from build123d import *

# Parameters (mm, degrees)
EXTRUDE_1_DEPTH             = 112
CUT_EXTRUDE_2_DEPTH         = 122.893396048
HOLE_WIZARD_M61_D           = 6.6
HOLE_WIZARD_M61_DEPTH       = 20
HOLE_WIZARD_M61_CBORE_D     = 11
HOLE_WIZARD_M61_CBORE_DEPTH = 12.4
HOLE_WIZARD_M61_TIP         = 1.982840043


with BuildPart() as part:
    # Эскиз1 → Бобышка-Вытянуть1 (new, symmetric)
    with BuildSketch(Plane.XY):
        Polygon((22.5, 0), (-22.5, 0), (-22.5, 10.4), (-7.5, 10.4), (-7.5, 17), (7.5, 17), (7.5, 10.4), (22.5, 10.4), align=None)
    extrude(amount=EXTRUDE_1_DEPTH, both=True)

    # Эскиз5 → Вырез-Вытянуть2 (cut, through all)
    with BuildSketch(Plane(origin=(22.5, 0, 0), x_dir=(0, 0, -1), z_dir=(1, 0, 0))):
        Polygon((-112, 0), (-48.555136271, 17), (-112, 17), align=None)
    extrude(amount=-CUT_EXTRUDE_2_DEPTH, mode=Mode.SUBTRACT)

    # Цековка для винта с внутренним шестигранником M61
    with Locations(Plane(origin=(0, 17, 0), x_dir=(1, 0, 0), z_dir=(0, 1, 0))):
        with Locations((0, -210), (0, 70), (0, -70)):
            CounterBoreHole(HOLE_WIZARD_M61_D / 2, HOLE_WIZARD_M61_CBORE_D / 2, HOLE_WIZARD_M61_CBORE_DEPTH, depth=HOLE_WIZARD_M61_DEPTH)
            with Locations((0, 0, -(HOLE_WIZARD_M61_DEPTH + HOLE_WIZARD_M61_TIP / 2))):  # 118° drill point
                Cone(0, HOLE_WIZARD_M61_D / 2, HOLE_WIZARD_M61_TIP, mode=Mode.SUBTRACT)


solid = part.part
The listing builds one solid part. Answer for the finished solid, in the listing's coordinates (mm). A direction names the side the tool comes from. Round coordinates to 2 decimals unless told otherwise and drop trailing zeros. Order: outer loops, then holes, each group sorted by start corner. A loop starts at its lowest first (then second) coordinate and runs counter-clockwise, first axis right, second up. Notation, with made-up numbers: M 6,5 L 61,5 A31 ccw 61,35 Z; hole C 4.5,13.25 d10. An arc over 180 degrees is marked long. Answer in a Markdown table with one row per item. Add a question column.
1) Consider line 1 along X through (y, z) = (10, 70); line 2 along X through (y, z) = (3.25, -70); line 3 along Y through (x, z) = (-11.5, -55). Determine where each line is inside the solid, lowest interval first. Write a range as from..to.
2) The part is cut by section B-B on x = 0. Determine the outline of the cut face in (y, z).
3) The part is cut by section C-C on z = 27.5. Determine the outline of the cut face in (x, y).
4) Flat-ended cylindrical pins translate along their axes: pin 1 Ø12 at (x, z) = (-1.5, 69.5) entering from +Y; pin 2 Ø12 at (x, z) = (-15.5, 16.5) entering from +Y; pin 3 Ø7.5 at (x, z) = (0, 70) entering from +Y; pin 4 Ø4 at (x, z) = (0, -70) entering from +Y. Find the tip coordinate at first contact, or state that the pin passes through.
5) Which of the six approach directions +Z, -Z, +X, -X, +Y, -Y give full straight-line access (tool end or side, diameter ignored) to faces 1 (the face through (7.5, 14, -18)), 2 (the face through (2.957, 7.832, 65.362)), 3 (the face through (0.315, 6.492, 87.771)), 4 (the face through (-7.5, 14, -18))?
6) The part is cut by section D-D on y = 2.75. Determine the outline of the cut face in (x, z).
7) The part is cut by section A-A on z = -70. Determine the outline of the cut face in (x, y).
8) Determine the mould class of faces 5 (the face through (0, 17, -31)), 6 (the face through (-0.716, 10.887, -75.453)), 7 (the face through (0, 7, -112)) for opening direction Z: pulls with the +Z half, pulls with the -Z half, needs draft (parallel to the pull), parting line crosses it, or undercut.
Findings below:
| question | item | result |
|---|---|---|
| 1 | line 1 | x = -22.5..-5.5, 5.5..22.5 |
| 1 | line 2 | x = -22.5..-3.3, 3.3..22.5 |
| 1 | line 3 | y = 0..10.4 |
| 2 | outline | M 0,-112 L 17,-112 L 17,-75.5 L 4.6,-75.5 L 4.6,-73.3 L 0,-73.3 Z; M 0,-66.7 L 4.6,-66.7 L 4.6,-64.5 L 17,-64.5 L 17,48.56 L 12.73,64.5 L 4.6,64.5 L 4.6,66.7 L 0,66.7 Z; M 0,73.3 L 4.6,73.3 L 4.6,75.5 L 9.78,75.5 L 0,112 Z |
| 3 | outline | M -22.5,0 L 22.5,0 L 22.5,10.4 L 7.5,10.4 L 7.5,17 L -7.5,17 L -7.5,10.4 L -22.5,10.4 Z |
| 4 | pin 1 | stops at y = 13 |
| 4 | pin 2 | stops at y = 10.4 |
| 4 | pin 3 | stops at y = 4.6 |
| 4 | pin 4 | passes through |
| 5 | face 1 | +Z, -Z, +X, +Y |
| 5 | face 2 | +Y |
| 5 | face 3 | +Z, +X, -X, +Y |
| 5 | face 4 | +Z, -Z, -X, +Y |
| 6 | outline | M -22.5,-112 L 22.5,-112 L 22.5,101.74 L -22.5,101.74 Z; hole C 0,-70 d6.6; hole C 0,70 d6.6 |
| 7 | outline | M -22.5,0 L -3.3,0 L -3.3,4.6 L -5.5,4.6 L -5.5,17 L -7.5,17 L -7.5,10.4 L -22.5,10.4 Z; M 3.3,0 L 22.5,0 L 22.5,10.4 L 7.5,10.4 L 7.5,17 L 5.5,17 L 5.5,4.6 L 3.3,4.6 Z |
| 8 | face 5 | needs draft |
| 8 | face 6 | undercut |
| 8 | face 7 | pulls with the -Z half |
